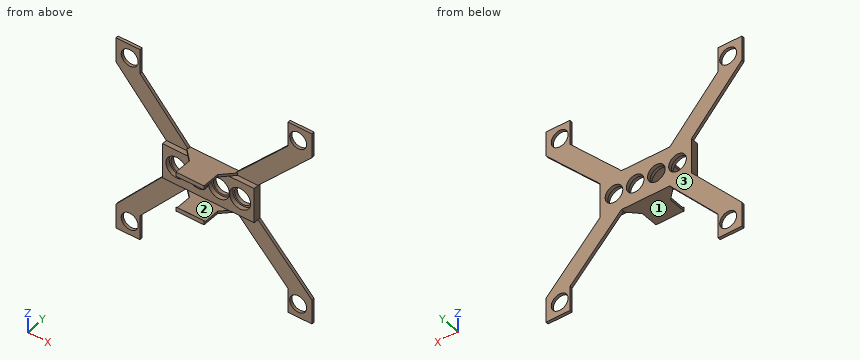
from build123d import *

# Parameters (mm, degrees)
SKICA1_W                 = 26
SKICA1_H                 = 1
P_IDAT_VYSUNUT_M1_DEPTH  = 10
SKICA2_R                 = 2.5
ODEBRAT_VYSUNUT_M1_DEPTH = 1
SKICA3_R                 = 2.4
P_IDAT_VYSUNUT_M2_DEPTH  = 0.8
SKICA4_W                 = 26
SKICA4_H                 = 10
SKICA4_R                 = 3
P_IDAT_VYSUNUT_M3_DEPTH  = 1.2
SKICA6_W                 = 8
SKICA6_H                 = 0.7
P_IDAT_VYSUNUT_M5_DEPTH  = 9
P_IDAT_VYSUNUT_M6_DEPTH  = 8
P_IDAT_VYSUNUT_M8_DEPTH  = 0.7
P_IDAT_VYSUNUT_M9_DEPTH  = 0.7


with BuildPart() as part:
    # Skica1 → Přidat vysunutím1 (new body)
    with BuildSketch(Plane.XY):
        with Locations((-39.156744291, -7.214704976)):
            Rectangle(SKICA1_W, SKICA1_H)
    extrude(amount=P_IDAT_VYSUNUT_M1_DEPTH)

    # Skica2 → Odebrat vysunutím1 (cut)
    with BuildSketch(Plane(origin=(0, -7.714704976, 0), x_dir=(-1, 0, 0), z_dir=(0, -1, 0))):
        with Locations((48.186744291, -5)):
            Circle(SKICA2_R)
        with Locations((42.176744291, -5)):
            Circle(SKICA2_R)
        with Locations((36.166744291, -5)):
            Circle(SKICA2_R)
        with Locations((30.156744291, -5)):
            Circle(SKICA2_R)
    extrude(amount=-ODEBRAT_VYSUNUT_M1_DEPTH, mode=Mode.SUBTRACT)

    # Skica3 → Přidat vysunutím2 (add)
    with BuildSketch(Plane(origin=(0, -6.714704976, 0), x_dir=(1, 0, 0), z_dir=(0, 1, 0))):
        Polygon((-32.956744291, 0), (-17.656744291, 15.8), (-17.656744291, 22.8), (-10.856744291, 22.8), (-10.856744291, 15.8), (-26.156744291, 0), align=None)
        with Locations((-14.756744291, 18.9)):
            Circle(SKICA3_R, mode=Mode.SUBTRACT)
        Polygon((-52.156744291, 0), (-45.356744291, 0), (-59.656744291, 15.8), (-59.656744291, 22.8), (-66.456744291, 22.8), (-66.456744291, 15.8), align=None)
        with Locations((-62.556744291, 18.9)):
            Circle(SKICA3_R, mode=Mode.SUBTRACT)
        Polygon((-45.356744291, -10), (-59.656744291, -25.8), (-59.656744291, -32.8), (-66.456744291, -32.8), (-66.456744291, -25.8), (-52.156744291, -10), align=None)
        with Locations((-62.556744291, -28.9)):
            Circle(SKICA3_R, mode=Mode.SUBTRACT)
        Polygon((-26.156744291, -10), (-32.956744291, -10), (-17.656744291, -25.8), (-17.656744291, -32.8), (-10.856744291, -32.8), (-10.856744291, -25.8), align=None)
        with Locations((-14.756744291, -28.9)):
            Circle(SKICA3_R, mode=Mode.SUBTRACT)
    extrude(amount=-P_IDAT_VYSUNUT_M2_DEPTH)

    # Skica4 → Přidat vysunutím3 (add)
    with BuildSketch(Plane(origin=(0, -7.714704976, 0), x_dir=(-1, 0, 0), z_dir=(0, -1, 0))):
        with Locations((39.156744291, -5)):
            Rectangle(SKICA4_W, SKICA4_H)
        with Locations((48.186744291, -5)):
            Circle(SKICA4_R, mode=Mode.SUBTRACT)
        with Locations((42.176744291, -5)):
            Circle(SKICA4_R, mode=Mode.SUBTRACT)
        with Locations((36.166744291, -5)):
            Circle(SKICA4_R, mode=Mode.SUBTRACT)
        with Locations((30.156744291, -5)):
            Circle(SKICA4_R, mode=Mode.SUBTRACT)
    extrude(amount=P_IDAT_VYSUNUT_M3_DEPTH)

    # Skica6 → Přidat vysunutím5 (add)
    with BuildSketch(Plane(origin=(0, -6.714704976, 0), x_dir=(1, 0, 0), z_dir=(0, 1, 0))):
        with Locations((-39.156744291, 0.35)):
            Rectangle(SKICA6_W, SKICA6_H)
        with Locations((-39.156744291, -10.35)):
            Rectangle(SKICA6_W, SKICA6_H)
    extrude(amount=-P_IDAT_VYSUNUT_M5_DEPTH)

    # Skica7 → Přidat vysunutím6 (add)
    with BuildSketch(Plane(origin=(-35.156744291, 0, 0), x_dir=(0, 0, -1), z_dir=(1, 0, 0))):
        Polygon((-10, -15.714704976), (-9.5, -15.714704976), (-10, -15.214704976), align=None)
        Polygon((0, -15.714704976), (0, -15.214704976), (-0.5, -15.714704976), align=None)
    extrude(amount=-P_IDAT_VYSUNUT_M6_DEPTH)

    # Skica8 → Přidat vysunutím8 (add)
    with BuildSketch(Plane(origin=(0, 0, 0), x_dir=(-1, 0, 0), z_dir=(0, 0, -1))):
        Polygon((43.156744291, -6.714704976), (43.156744291, -10.714704976), (47.156744291, -6.714704976), align=None)
        Polygon((35.156744291, -10.714704976), (35.156744291, -6.714704976), (31.156744291, -6.714704976), align=None)
    extrude(amount=P_IDAT_VYSUNUT_M8_DEPTH)

    # Skica9 → Přidat vysunutím9 (add)
    with BuildSketch(Plane.XY.offset(10)):
        Polygon((-43.156744291, -6.714704976), (-47.156744291, -6.714704976), (-43.156744291, -10.714704976), align=None)
        Polygon((-35.156744291, -6.714704976), (-35.156744291, -10.714704976), (-31.156744291, -6.714704976), align=None)
    extrude(amount=P_IDAT_VYSUNUT_M9_DEPTH)


solid = part.part
The listing builds one solid part. Answer for the finished solid, in the listing's coordinates (mm). Face numbers are marked on the shaded views. Give positions to 0.01 mm unless a question says otherwise; leave off trailing zeros. Order: outer loops, then holes, each group sorted by start corner. A loop starts at its lowest first (then second) coordinate and runs counter-clockwise, first axis right, second up. Notation, with made-up numbers: (31, 41.25) - (82, 41.25) arc R16 ccw to (82, 56.25) - close; hole circle Ø10 at (40, 69.25). An arc over 180 degrees is marked (long way). Use one line per item in the form item = value.
1) Consider probe 1 along X at (y, z) = (-7.15, 5); probe 2 along X at (y, z) = (-7.3, -18.9); probe 3 along Z at (x, y) = (-37, -9.25). Determine where each line is inside the solid, lowest interval first. Write a range as [from, to].
Verdict:
probe_1 = [-52.16, -50.69], [-45.69, -44.68], [-39.68, -38.67], [-33.67, -32.66], [-27.66, -26.16]
probe_2 = [-66.46, -64.96], [-60.16, -59.66], [-17.66, -17.16], [-12.36, -10.86]
probe_3 = [-0.7, 0], [10, 10.7]
2) Find section A-A on y = -13.5. Determine the outline of the cut face in (x, z), and give its area (3 significant figures).
Verdict:
outline = (-43.16, -0.7) - (-35.16, -0.7) - (-35.16, 0) - (-43.16, 0) - close; (-43.16, 10) - (-35.16, 10) - (-35.16, 10.7) - (-43.16, 10.7) - close
area = 11.2 mm^2
3) Each of these flat-tipped pins is pushed along its axis until it touches: pin 1 (1.8 mm diameter, centred on x = -48, z = 4.5, fed in from -Y); pin 2 (4.5 mm diameter, centred on x = -40.5, y = -11.5, fed in from +Z); pin 3 (0.7 mm diameter, centred on x = -31, y = -8.5, fed in from -Z); pin 4 (1.3 mm diameter, centred on y = -12.5, z = 10.5, fed in from -X). Where does it stop, or does it pass through?
Verdict:
pin_1 = through
pin_2 = 10.7
pin_3 = 0
pin_4 = -43.16
4) Find section B-B on z = 28.9. Determine the outline of the cut face in (x, y), and give its area (3 significant figures).
Verdict:
outline = (-66.46, -7.51) - (-64.96, -7.51) - (-64.96, -6.71) - (-66.46, -6.71) - close; (-60.16, -7.51) - (-59.66, -7.51) - (-59.66, -6.71) - (-60.16, -6.71) - close; (-17.66, -7.51) - (-17.16, -7.51) - (-17.16, -6.71) - (-17.66, -6.71) - close; (-12.36, -7.51) - (-10.86, -7.51) - (-10.86, -6.71) - (-12.36, -6.71) - close
area = 3.20 mm^2
5) The mould has two halves that part along Z. Classify the marked faces 1, 2 and 3: released by +Z, released by -Z, zero draft, split by the parting line, or undercut.
Verdict:
face_1 = released by -Z
face_2 = undercut
face_3 = zero draft
6) Find section D-D on z = -11.5. Determine the outline of the cut face in (x, y).
Verdict:
outline = (-62.56, -7.51) - (-55.76, -7.51) - (-55.76, -6.71) - (-62.56, -6.71) - close; (-21.82, -7.51) - (-15.02, -7.51) - (-15.02, -6.71) - (-21.82, -6.71) - close
7) Find section C-C on x = -28.5. Determine the outline of the cut face in (y, z), and give its area (3 significant figures).
Verdict:
outline = (-8.91, 0) - (-7.51, 0) - (-7.51, -4.6) - (-6.71, -4.6) - (-6.71, 3.13) - (-7.71, 3.13) - (-7.71, 2.5) - (-8.91, 2.5) - close; (-8.91, 7.5) - (-7.71, 7.5) - (-7.71, 6.87) - (-6.71, 6.87) - (-6.71, 14.6) - (-7.51, 14.6) - (-7.51, 10) - (-8.91, 10) - close
area = 19.6 mm^2
